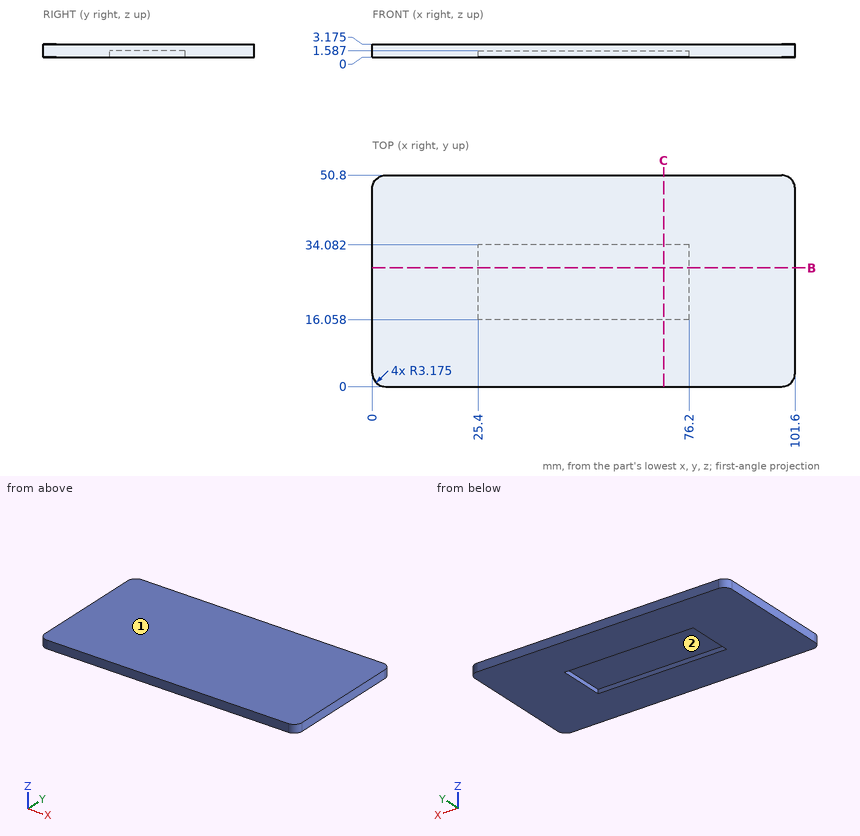
Print and shaded views of the part. All mm, measured from the part's lowest x, y and z. Coordinates: 2 decimals unless noted, no trailing zeros. Order: outer loops, then holes, each group sorted by start corner. A loop starts at its lowest first (then second) coordinate and runs counter-clockwise, first axis right, second up. Notation, with made-up numbers: (-6, 48.25) -> (33, 48.25) arc R21 cw to (33, 84.25) -> close; hole circle Ø5 at (35, 75.5). An arc over 180 degrees is marked (long way). Answer as a JSON object with one key per item and string values. Group by question number.
1) Flat gauge pin, fed straight in: pin 1 (9 mm diameter, centred on x = 57.5, y = 26, fed in from -Z). Where does the tip first touch, or does it go through?
2) Pull direction X, two halves, no side cores. Call the marked faces 1 and 2: +X half, -X half, draft (parallel to the pull), parting line (faces both ways), or undercut.
3) Drill centre lines: L1, parallel to X at y = 24, z = 0.7; L2, parallel to Y at x = 71, z = 0.6; L3, parallel to X at y = 48, z = 2.3. Where is each one in solid material? Low to high.
4) Cut at B-B, the plane y = 28.5. Write the cut outline in (x, z) (1 decimal), then the cut area to 3 significant figures.
5) Cut at C-C, the plane x = 70. Write the cut outline in (y, z) (1 decimal), then the cut area to 3 significant figures.
Check values:
{
 "1": {"pin 1": "stops at z = 1.59"},
 "2": {"face 1": "draft", "face 2": "undercut"},
 "3": {"L1": "x = 0 to 25.4, 76.2 to 101.6", "L2": "y = 0 to 16.06, 34.08 to 50.8", "L3": "x = 0.02 to 101.58"},
 "4": {"outline": "(0, 0) -> (25.4, 0) -> (25.4, 1.6) -> (76.2, 1.6) -> (76.2, 0) -> (101.6, 0) -> (101.6, 3.2) -> (0, 3.2) -> close", "area": "242 mm²"},
 "5": {"outline": "(0, 0) -> (16.1, 0) -> (16.1, 1.6) -> (34.1, 1.6) -> (34.1, 0) -> (50.8, 0) -> (50.8, 3.2) -> (0, 3.2) -> close", "area": "133 mm²"}
}
